Source: CAD feature listing. Evaluate the final solid. Frame: model axes, mm. Give positions to 0.01 mm unless a question says otherwise; leave off trailing zeros. Order: outer loops, then holes, each group sorted by start corner. A loop starts at its lowest first (then second) coordinate and runs counter-clockwise, first axis right, second up.
from build123d import *

# Parameters (mm, degrees)
BOSS_EXTRUDE1_DEPTH                         = 101.6
SKETCH2_R                                   = 1.5875
CUT_EXTRUDE1_DEPTH                          = 101.6
CBORE_FOR_10_SOCKET_HEAD_CAP_SCREW2_OUT_R   = 2.5527
CBORE_FOR_10_SOCKET_HEAD_CAP_SCREW2_OUT_R_2 = 1.5875
CBORE_FOR_10_SOCKET_HEAD_CAP_SCREW2_DEPTH   = 101.6


# Read off the part's stored shape, not the designer's step: CBORE for #10 Socket Head Cap Screw2
with BuildPart() as part:
    # Sketch1 → Boss-Extrude1 (new body)
    with BuildSketch(Plane.XY):
        with BuildLine():
            Line((-4.70551159, -4.549815043), (-3.666174521, -6.349999904))
            Line((-3.666174521, -6.349999904), (-1.587501923, -6.349999904))
            ThreePointArc((-1.587501923, -6.349999904), (-3.85e-07, -4.762498365), (1.587501923, -6.349999904))
            Line((1.587501923, -6.349999904), (3.666173825, -6.349999904))
            Line((3.666173825, -6.349999904), (4.705510929, -4.549815232))
            ThreePointArc((4.705510929, -4.549815232), (4.124445601, -2.381249904), (6.293010929, -1.800184575))
            Line((6.293010929, -1.800184575), (7.332348034, 9.6e-08))
            Line((7.332348034, 9.6e-08), (6.293011178, 1.800184715))
            ThreePointArc((6.293011178, 1.800184715), (4.124445902, 2.381250241), (4.705511428, 4.549815516))
            Line((4.705511428, 4.549815516), (3.666174521, 6.350000222))
            Line((3.666174521, 6.350000222), (1.587498077, 6.350000222))
            ThreePointArc((1.587498077, 6.350000222), (3.85e-07, 4.76250253), (-1.587498077, 6.350000222))
            Line((-1.587498077, 6.350000222), (-3.666173825, 6.350000222))
            Line((-3.666173825, 6.350000222), (-4.705511038, 4.549815614))
            ThreePointArc((-4.705511038, 4.549815614), (-4.124445841, 2.38125025), (-6.293011205, 1.800185053))
            Line((-6.293011205, 1.800185053), (-7.332348419, 4.44e-07))
            Line((-7.332348419, 4.44e-07), (-6.293011423, -1.80018429))
            ThreePointArc((-6.293011423, -1.80018429), (-4.12444613, -2.38124975), (-4.70551159, -4.549815043))
        make_face()
    extrude(amount=BOSS_EXTRUDE1_DEPTH)

    # Sketch2 → Cut-Extrude1 (cut)
    with BuildSketch(Plane.XY.offset(101.6)):
        Circle(SKETCH2_R)
    extrude(amount=-CUT_EXTRUDE1_DEPTH, mode=Mode.SUBTRACT)

    # CBORE for #10 Socket Head Cap Screw2 out → CBORE for #10 Socket Head Cap Screw2 (cut)
    with BuildSketch(Plane.XY):
        Circle(CBORE_FOR_10_SOCKET_HEAD_CAP_SCREW2_OUT_R)
        Circle(CBORE_FOR_10_SOCKET_HEAD_CAP_SCREW2_OUT_R_2, mode=Mode.SUBTRACT)
    extrude(amount=CBORE_FOR_10_SOCKET_HEAD_CAP_SCREW2_DEPTH, mode=Mode.SUBTRACT)


solid = part.part
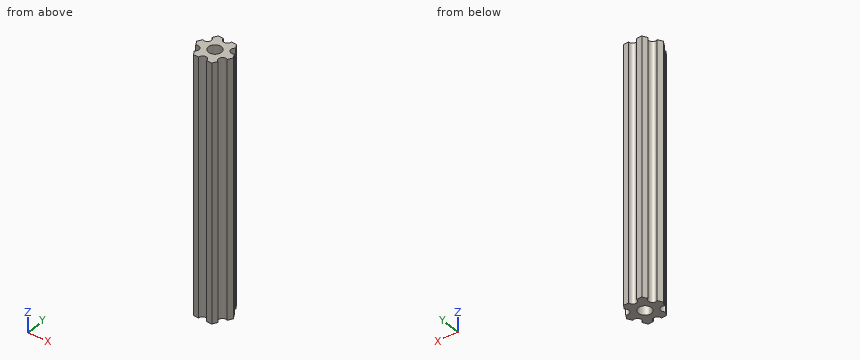
1) Section query A-A on x = 0. Output: boundary loops of the cut face in (y, z).
Checks:
outline: (-4.76, 0) - (-2.55, 0) - (-2.55, 101.6) - (-4.76, 101.6) - close; (2.55, 0) - (4.76, 0) - (4.76, 101.6) - (2.55, 101.6) - close
2) First-contact query: pin 1 Ø1 at (y, z) = (-2.5, 16.5) entering from +X; pin 2 Ø6 at (y, z) = (-2, 64) entering from +X; pin 3 Ø2 at (y, z) = (-1.5, 52) entering from -X. Flat tips, straight axial feed; report the tip coordinate or a pass-through.
Checks:
pin 1: stops at x = 4.43
pin 2: stops at x = 7.33
pin 3: stops at x = -7.04
3) Ray query, L1, parallel to Y at x = 0, z = 58.5; L2, parallel to Y at x = -4.25, z = 67; L3, parallel to Y at x = 4.5, z = 16. Return the intervals inside material, ascending.
Checks:
L1: y = -4.76 to -2.55, 2.55 to 4.76
L2: y = -5.34 to -4.15, -2.2 to 2.2, 4.15 to 5.34
L3: y = -4.91 to -4.41, -1.94 to 1.94, 4.41 to 4.91
